The listing builds one solid part. Answer for the finished solid, in the listing's coordinates (mm). A direction names the side the tool comes from. Coordinates: 2 decimals unless noted, no trailing zeros. Loops run counter-clockwise (first coordinate to the right, second up) from the corner with the lowest first, then second, coordinate; pieces in that order, holes last. Notation, with made-up numbers: M 20.5,8.5 L 33.5,8.5 A27 cw 33.5,35.5 Z; hole C 48.25,-32.5 d4. An arc over 180 degrees is marked long. Return JSON: item names as keys, results as strings. Group by question number.
1. The mould has two halves that part along X. Classify faces 4 (the face through (25, 36, 1)), 5 (the face through (22, 32, 50)), 6 (the face through (22.042, 21.992, -38.381)), 7 (the face through (22, 73, -50)): pulls with the +X half, pulls with the -X half, needs draft (parallel to the pull), parting line crosses it, or undercut.
2. Section C-C (x = 13) is taken. Write down the section's boundary in (y, z), then the cut area to 3 significant figures.
3. Section A-A (z = -28) is taken. Write down the section's boundary in (x, y).
4. Which of the six approach directions +Z, -Z, +X, -X, +Y, -Y give full straight-line access (tool end or side, diameter ignored) to faces 1 (the face through (-20.5, 3, 39.9)), 2 (the face through (22, 34, 40)), 3 (the face through (22, 71, -40))?
5. Section D-D (y = 56.5) is taken. Write down the section's boundary in (x, z).
6. Given P1, Ø6, axis at y = 44, z = -41, coming from the +X side; P2, Ø3.5, axis at x = 22, y = 34, coming from the +Z side; P3, Ø1.5, axis at y = 13.5, z = 33.5, coming from the -X side; P4, Ø4, axis at x = -3.5, z = -32.5, coming from the +Y side, each flat-ended and moving along its own axis, determine where each tip first touches the part or whether it passes through.
7. Section B-B (z = 50) is taken. Write down the section's boundary in (x, y), then the cut area to 3 significant figures.
8. Straight lines are drawn through the part: L1, parallel to X at y = 2.15, z = -40; L2, parallel to Y at x = 22, z = -50.5; L3, parallel to Y at x = 22.5, z = 41. For each, find the intervals that lie inside material, in ascending order. Write a range as from..to.
```python
from build123d import *

# Parameters (mm, degrees)
SKETCH_1_W          = 44
SKETCH_1_H          = 120
EXTRUDE_1_DEPTH     = 6
SKETCH_1_3_W        = 6
SKETCH_1_3_H        = 120
EXTRUDE_2_DEPTH     = 74
SKETCH_2_R          = 13
SKETCH_2_R_2        = 3
CUT_EXTRUDE_1_DEPTH = 7
SKETCH_3_R          = 2.5
CUT_EXTRUDE_2_DEPTH = 10
SKETCH_4_R          = 2
CUT_EXTRUDE_3_DEPTH = 20
SKETCH_5_R          = 3.3
CUT_EXTRUDE_4_DEPTH = 10


with BuildPart() as part:
    # 草图1 → 凸台-拉伸1 (new body)
    with BuildSketch(Plane(origin=(0, 0, 0), x_dir=(1, 0, 0), z_dir=(0, 1, 0))):
        with Locations((-3, 0)):
            Rectangle(SKETCH_1_W, SKETCH_1_H)
    extrude(amount=EXTRUDE_1_DEPTH)

    # 草图1<3> → 凸台-拉伸2 (add)
    with BuildSketch(Plane(origin=(0, 0, 0), x_dir=(1, 0, 0), z_dir=(0, 1, 0))):
        with Locations((22, 0)):
            Rectangle(SKETCH_1_3_W, SKETCH_1_3_H)
    extrude(amount=EXTRUDE_2_DEPTH)

    # 草图2 → 切除-拉伸1 (cut, through all)
    with BuildSketch(Plane.ZY.offset(-19)):
        with Locations((0, 49.5)):
            Circle(SKETCH_2_R)
        with Locations((-28, 49.5)):
            Circle(SKETCH_2_R_2)
        with Locations((28, 49.5)):
            Circle(SKETCH_2_R_2)
    extrude(amount=-CUT_EXTRUDE_1_DEPTH, mode=Mode.SUBTRACT)

    # 草图3 → 切除-拉伸2 (cut)
    with BuildSketch(Plane(origin=(0, 6, 0), x_dir=(1, 0, 0), z_dir=(0, 1, 0))):
        with Locations((-18, 40)):
            Circle(SKETCH_3_R)
        with Locations((12, 40)):
            Circle(SKETCH_3_R)
        with Locations((-18, -40)):
            Circle(SKETCH_3_R)
        with Locations((12, -40)):
            Circle(SKETCH_3_R)
    extrude(amount=-CUT_EXTRUDE_2_DEPTH, mode=Mode.SUBTRACT)

    # 草图4 → 切除-拉伸3 (cut)
    with BuildSketch(Plane(origin=(0, 0, -60), x_dir=(-1, 0, 0), z_dir=(0, 0, -1))):
        with Locations((-22, 34)):
            Circle(SKETCH_4_R)
        with Locations((-22, 71)):
            Circle(SKETCH_4_R)
    cut_extrude_3 = extrude(amount=-CUT_EXTRUDE_3_DEPTH, mode=Mode.SUBTRACT)

    # 镜向1: 切除-拉伸3 across plane
    add(cut_extrude_3.mirror(Plane(origin=(0, 0, 0), x_dir=(1, 0, 0), z_dir=(0, 0, -1))), mode=Mode.SUBTRACT)

    # 草图5 → 切除-拉伸4 (cut)
    with BuildSketch(Plane(origin=(25, 0, 0), x_dir=(0, 0, -1), z_dir=(1, 0, 0))):
        with Locations((41, 44)):
            Circle(SKETCH_5_R)
        with Locations((41, 24)):
            Circle(SKETCH_5_R)
        with Locations((-41, 24)):
            Circle(SKETCH_5_R)
        with Locations((-41, 44)):
            Circle(SKETCH_5_R)
    extrude(amount=-CUT_EXTRUDE_4_DEPTH, mode=Mode.SUBTRACT)


solid = part.part
```
Worked out:
{
 "1": {"face 4": "pulls with the +X half", "face 5": "undercut", "face 6": "needs draft", "face 7": "undercut"},
 "2": {"outline": "M 0,-60 L 6,-60 L 6,-42.29 L 0,-42.29 Z; M 0,-37.71 L 6,-37.71 L 6,37.71 L 0,37.71 Z; M 0,42.29 L 6,42.29 L 6,60 L 0,60 Z", "area": "665 mm^2"},
 "3": {"outline": "M -25,0 L 25,0 L 25,46.5 L 19,46.5 L 19,6 L -25,6 Z; M 19,52.5 L 25,52.5 L 25,74 L 19,74 Z"},
 "4": {"face 1": "+Y, -Y", "face 2": "+Z", "face 3": "-Z"},
 "5": {"outline": "M 19,-60 L 25,-60 L 25,-10.95 L 19,-10.95 Z; M 19,10.95 L 25,10.95 L 25,60 L 19,60 Z"},
 "6": {"P1": "through", "P2": "z = 40", "P3": "x = 19", "P4": "y = 6"},
 "7": {"outline": "M -25,0 L 25,0 L 25,74 L 19,74 L 19,6 L -25,6 Z; hole C 22,34 d4; hole C 22,71 d4", "area": "683 mm^2"},
 "8": {"L1": "-25..-20.5, -15.5..9.5, 14.5..25", "L2": "0..32, 36..69, 73..74", "L3": "0..20.7, 27.3..32.06, 35.94..40.7, 47.3..69.06, 72.94..74"}
}
